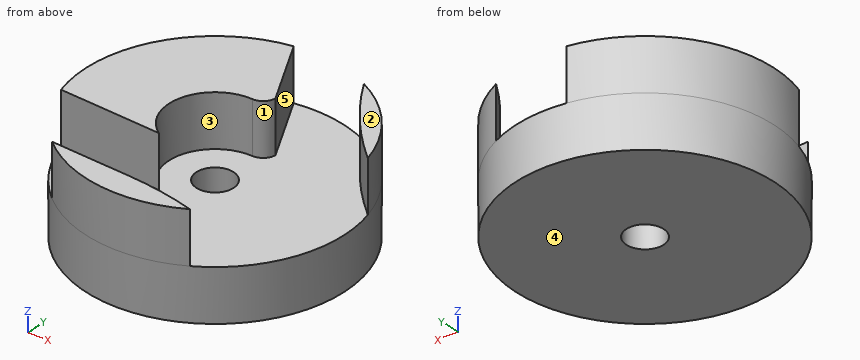
from build123d import *

# Parameters (mm, degrees)
CROQUIS2_R              = 15
SALIENTE_EXTRUIR1_DEPTH = 6
CROQUIS3_R              = 2.159
CORTAR_EXTRUIR1_DEPTH   = 6
SALIENTE_EXTRUIR2_DEPTH = 6


with BuildPart() as part:
    # Croquis2 → Saliente-Extruir1 (new body)
    with BuildSketch(Plane.XY):
        with Locations((-0.424832659, 0)):
            Circle(CROQUIS2_R)
    extrude(amount=SALIENTE_EXTRUIR1_DEPTH)

    # Croquis3 → Cortar-Extruir1 (cut)
    with BuildSketch(Plane(origin=(0, 0, 0), x_dir=(-1, 0, 0), z_dir=(0, 0, -1))):
        with Locations((0.424832659, 0)):
            Circle(CROQUIS3_R)
    extrude(amount=-CORTAR_EXTRUIR1_DEPTH, mode=Mode.SUBTRACT)

    # Croquis5 → Saliente-Extruir2 (add)
    with BuildSketch(Plane.XY.offset(6)):
        with BuildLine():
            Line((1.150657303, 6.727260511), (-3.173951667, 14.745926376))
            ThreePointArc((-3.173951667, 14.745926376), (-13.192330391, 7.873436458), (-14.835285649, -4.16399383))
            Line((-14.835285649, -4.16399383), (-3.282721328, -4.499041271))
            ThreePointArc((-3.282721328, -4.499041271), (-5.537081833, 1.507915241), (-0.38358243, 5.329840374))
            ThreePointArc((-0.38358243, 5.329840374), (0.657157734, 5.728140337), (1.150657303, 6.727260511))
        make_face()
        with BuildLine():
            ThreePointArc((14.060690832, 3.894818251), (11.020642477, 9.695416387), (5.798891595, 13.647903004))
            ThreePointArc((5.798891595, 13.647903004), (9.512311917, 8.417715579), (14.060690832, 3.894818251))
        make_face()
        with BuildLine():
            Line((-0.730311074, -11.926156717), (-9.859444413, -11.661393616))
            ThreePointArc((-9.859444413, -11.661393616), (-1.589548178, -14.954712895), (7.090520152, -12.981505003))
            ThreePointArc((7.090520152, -12.981505003), (3.207869051, -12.248077397), (-0.730311074, -11.926156717))
        make_face()
    extrude(amount=SALIENTE_EXTRUIR2_DEPTH)


solid = part.part
Can you work these out from the model? Positions are in its coordinate system, mm. Face numbers are marked on the shaded views. A direction names the side the tool comes from. Coordinates: 2 decimals unless noted, no trailing zeros. Loops run counter-clockwise (first coordinate to the right, second up) from the corner with the lowest first, then second, coordinate; pieces in that order, holes last. Notation, with made-up numbers: M 26.25,68.5 L 72.25,68.5 A20 ccw 72.25,83.5 Z; hole C 27.5,24 d11. An arc over 180 degrees is marked long. Return JSON: item names as keys, results as strings. Group by question number.
Item 1: On a 3-axis mill with a long thin cutter (end or side, diameter ignored), from which of +Z, -Z, +X, -X, +Y, -Y can I reach the whole of each face in a straight line? I mean the marked faces 1 and 2. Say none if no direction works.
Item 2: If I drill on L1, parallel to Y at x = -4, z = 7.5; L2, parallel to Z at x = -2, y = -4; L3, parallel to X at y = -1.5, z = 4.5, over which ranges is the centre line in solid material (lowest first)? Write a range as from..to.
Item 3: Imagine slicing it at B-B (z = 6.75). Please give me the cut outline in (x, y).
Item 4: Imagine slicing it at C-C (x = -11.5). Please give me the cut outline in (y, z).
Item 5: I'm going to push flat-ended pins straight in: pin 1 Ø3 at (x, z) = (-12.5, 3) entering from -Y; pin 2 Ø1.5 at (x, z) = (-6, 7) entering from -Y; pin 3 Ø4 at (x, z) = (8.5, 2.5) entering from +Y; pin 4 Ø4 at (x, y) = (-0.42, 0) entering from -Z. Where does each tip first touch, or does it pass through?
Item 6: Imagine slicing it at D-D (x = 2.5). Please give me the cut outline in (y, z), and give its area (3 significant figures).
Item 7: Imagine slicing it at A-A (y = 0). Please give me the cut outline in (x, z), and give its area (3 significant figures).
Item 8: Thinking about a two-plate mould opening in Y: for the marked faces 3, 4 and 5, which applies, released by +Y, released by -Y, zero draft, split by the parting line, or undercut?
Verdict:
{
 "1": {"face 1": "+Z", "face 2": "+Z, +X, -X, +Y, -Y"},
 "2": {"L1": "y = -14.57..-11.83, -4.48..-3.95, 3.95..14.57", "L2": "z = 0..6", "L3": "x = -15.35..-1.98, 1.13..14.5"},
 "3": {"outline": "M -14.84,-4.16 L -3.28,-4.5 A5.33 cw -0.38,5.33 A1.53 ccw 1.15,6.73 L -3.17,14.75 A15 ccw Z; M -9.86,-11.66 A15 ccw 7.09,-12.98 A37.6 ccw -0.73,-11.93 Z; M 5.8,13.65 A37.6 ccw 14.06,3.89 A15 ccw Z"},
 "4": {"outline": "M -10.12,0 L 10.12,0 L 10.12,12 L -4.26,12 L -4.26,6 L -10.12,6 Z"},
 "5": {"pin 1": "stops at y = -10.64", "pin 2": "stops at y = -14.2", "pin 3": "stops at y = 13.31", "pin 4": "passes through"},
 "6": {"outline": "M -14.71,0 L 14.71,0 L 14.71,6 L -12.16,6 L -12.16,12 L -14.71,12 Z", "area": "192 mm^2"},
 "7": {"outline": "M -15.42,0 L -2.58,0 L -2.58,6 L -5.75,6 L -5.75,12 L -15.42,12 Z; M 1.73,0 L 14.58,0 L 14.58,6 L 1.73,6 Z", "area": "212 mm^2"},
 "8": {"face 3": "undercut", "face 4": "zero draft", "face 5": "released by +Y"}
}
